from build123d import *

# Parameters (mm, degrees)
F1_DEPTH = 100
F2_W     = 5
F2_H     = 581
F2_W_2   = 1636.7888212204
F2_H_2   = 5
F2_W_3   = 600
F2_H_3   = 1200
F2_W_4   = 607.3750638962
F3_DEPTH = 25
F4_W     = 2650
F4_H     = 5
F5_DEPTH = 25


with BuildPart() as f1:
    # F0 (on Right) → F1 (new body)
    with BuildSketch(Plane.YZ):
        Polygon((389.0280389786, 767.0902125925), (389.0280389786, 33.4885828197), (1817.3750638962, 33.4885828197), (1817.3750638962, 1807.9981070012), align=None)
    extrude(amount=-F1_DEPTH)

    # F2 (on Right) → F3 (cut)
    with BuildSketch(Plane.YZ):
        with Locations((1214.8750638962, 1528.9885828197)):
            Rectangle(F2_W, F2_H)
        with Locations((2035.7694745064, 1235.9885828197)):
            Rectangle(F2_W_2, F2_H_2)
        with Locations((1214.8750638962, 1235.9885828197)):
            Rectangle(F2_W, F2_H_2)
        with Locations((912.3750638962, 1235.9885828197)):
            Rectangle(F2_W_3, F2_H_2)
        with Locations((1214.8750638962, 633.4885828197)):
            Rectangle(F2_W, F2_H_3)
        with Locations((609.8750638962, 1528.9885828197)):
            Rectangle(F2_W, F2_H)
        with Locations((609.8750638962, 1235.9885828197)):
            Rectangle(F2_W, F2_H_2)
        with Locations((609.8750638962, 633.4885828197)):
            Rectangle(F2_W, F2_H_3)
        with Locations((303.6875319481, 1235.9885828197)):
            Rectangle(F2_W_4, F2_H_2)
    extrude(amount=-F3_DEPTH, mode=Mode.SUBTRACT)

    # F4 (on face) → F5 (cut)
    with BuildSketch(Plane.YZ):
        with Locations((1624.0280389786, 785.9885828197)):
            Rectangle(F4_W, F4_H)
    extrude(amount=-F5_DEPTH, mode=Mode.SUBTRACT)


solid = f1.part
Verification items for the finished model (mm, model axes). Coordinates: 2 decimals unless noted, no trailing zeros. Write each loop counter-clockwise with the first axis right and the second up, starting at its lowest first coordinate (ties: lowest second). Pieces come first, ordered by that corner, then holes. Notation, with made-up numbers: M -13,-23 L 25,-23 A6 ccw 25,-17 Z; hole C 88.25,25.5 d9. An arc over 180 degrees is marked long. Use CSV: the item, a comma, the result in double quotes.
Q1. Section check B-B, the plane z = 1149.5. Enter the section's corners in (x, y), and give its area (3 significant figures).
Computed values:
outline,"M -100,913.78 L 0,913.78 L 0,1212.38 L -25,1212.38 L -25,1217.38 L 0,1217.38 L 0,1817.38 L -100,1817.38 Z"
area,"90,200 mm²"
Q2. Thickness scan on line 1 along Y through (x, z) = (-24, 572); line 2 along Z through (x, y) = (-23.5, 1409); line 3 along Z through (x, y) = (-31.5, 1213). Record the ranges inside material, lowest first. Write a range as [from, to].
Computed values:
line 1,"[389.03, 607.38], [612.38, 1212.38], [1217.38, 1817.38]"
line 2,"[33.49, 783.49], [788.49, 1233.49], [1238.49, 1510.39]"
line 3,"[33.49, 1367.56]"
Q3. Section check D-D, the plane z = 838. Enter the section's corners in (x, y).
Computed values:
outline,"M -100,486.33 L 0,486.33 L 0,607.38 L -25,607.38 L -25,612.38 L 0,612.38 L 0,1212.38 L -25,1212.38 L -25,1217.38 L 0,1217.38 L 0,1817.38 L -100,1817.38 Z"
Q4. Section check C-C, the plane x = -66. Enter the section's corners in (y, z), and give its area (3 significant figures).
Computed values:
outline,"M 389.03,33.49 L 1817.38,33.49 L 1817.38,1808 L 389.03,767.09 Z"
area,"1,790,000 mm²"
Q5. Go/stop test with flat-tipped pins: P1, Ø12.5, axis at x = -18.5, y = 532.5, coming from the +Z side; P2, Ø12.5, axis at x = -11.5, y = 1164, coming from the +Z side; P3, Ø12, axis at x = -23, y = 1097.5, coming from the +Z side. Record where each tip stops, or that it passes through.
Computed values:
P1,"z = 876.2"
P2,"z = 1336.41"
P3,"z = 1287.76"
Q6. Section check A-A, the plane y = 826. Enter the section's corners in (x, z), and give its area (3 significant figures).
Computed values:
outline,"M -100,33.49 L 0,33.49 L 0,783.49 L -25,783.49 L -25,788.49 L 0,788.49 L 0,1085.53 L -100,1085.53 Z"
area,"105,000 mm²"
